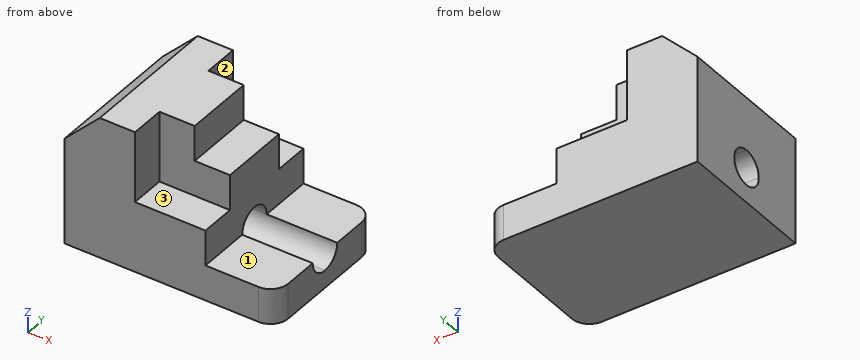
```python
from build123d import *

# Parameters (mm, degrees)
F0_W      = 76.2
F0_H      = 50.8
F1_DEPTH  = 50.8
F3_DEPTH  = 50.801
F5_DEPTH  = 12.7
F6_W      = 25.4
F6_H      = 25.4
F7_DEPTH  = 12.7
F9_DEPTH  = 12.701
F11_DEPTH = 76.201


with BuildPart() as f1:
    # F0 (on Front) → F1 (new body)
    with BuildSketch(Plane.XZ):
        with Locations((38.1, 25.4)):
            Rectangle(F0_W, F0_H)
    extrude(amount=F1_DEPTH)

    # F2 (on face) → F3 (cut, through all)
    with BuildSketch(Plane.XZ.offset(50.8)):
        Polygon((12.7, 50.8), (0, 50.8), (0, 38.1), align=None)
        Polygon((76.2, 12.7), (76.2, 50.8), (38.1, 50.8), (38.1, 38.1), (50.8, 38.1), (50.8, 12.7), align=None)
    extrude(amount=-F3_DEPTH, mode=Mode.SUBTRACT)

    # F4 (on face) → F5 (cut)
    with BuildSketch(Plane.XZ.offset(50.8)):
        Polygon((25.4, 50.8), (25.4, 25.4), (50.8, 25.4), (50.8, 38.1), (38.1, 38.1), (38.1, 50.8), align=None)
    extrude(amount=-F5_DEPTH, mode=Mode.SUBTRACT)

    # F6 (on face) → F7 (cut)
    with BuildSketch(Plane(origin=(0, 0, 0), x_dir=(-1, 0, 0), z_dir=(0, 1, 0))):
        with Locations((-38.1, 38.1)):
            Rectangle(F6_W, F6_H)
    extrude(amount=-F7_DEPTH, mode=Mode.SUBTRACT)

    # F8 (on face) → F9 (cut, through all)
    with BuildSketch(Plane.XY.offset(12.7)):
        with BuildLine():
            ThreePointArc((76.2, -44.45), (74.340128, -48.940128), (69.85, -50.8))
            Line((69.85, -50.8), (76.2, -50.8))
            Line((76.2, -50.8), (76.2, -44.45))
        make_face()
        with BuildLine():
            Line((76.2, 0), (69.85, 0))
            ThreePointArc((69.85, 0), (74.340128, -1.859872), (76.2, -6.35))
            Line((76.2, -6.35), (76.2, 0))
        make_face()
    extrude(amount=-F9_DEPTH, mode=Mode.SUBTRACT)

    # F10 (on face) → F11 (cut, through all)
    with BuildSketch(Plane.YZ.offset(76.2)):
        with BuildLine():
            ThreePointArc((-25.4, 6.35), (-20.909872, 8.209872), (-19.05, 12.7))
            ThreePointArc((-19.05, 12.7), (-20.909872, 17.190128), (-25.4, 19.05))
            ThreePointArc((-25.4, 19.05), (-29.890128, 17.190128), (-31.75, 12.7))
            ThreePointArc((-31.75, 12.7), (-29.890128, 8.209872), (-25.4, 6.35))
        make_face()
    extrude(amount=-F11_DEPTH, mode=Mode.SUBTRACT)


solid = f1.part
```
The listing builds one solid part. Answer for the finished solid, in the listing's coordinates (mm). Face numbers are marked on the shaded views. A direction names the side the tool comes from. Give positions to 0.01 mm unless a question says otherwise; leave off trailing zeros. Write each loop counter-clockwise with the first axis right and the second up, starting at its lowest first coordinate (ties: lowest second). Pieces come first, ordered by that corner, then holes. Notation, with made-up numbers: (10, 79.5) - (61, 79.5) arc R10 ccw to (61, 91.5) - close; hole circle Ø2 at (46.25, 51.5). An arc over 180 degrees is marked (long way). Use one line per item in the form item = value. Start each with the question number.
1) Consider line 1 along Z through (x, y) = (47.5, -5); line 2 along Y through (x, z) = (6.5, 8.5). Determine where each line is inside the solid, lowest interval first. Write a range as from..to.
2) Find section B-B on z = 41.5. Determine the outline of the cut face in (x, y).
3) Find section A-A on x = 23.5. Determine the outline of the cut face in (y, z), plus the area to 3 significant figures.
4) Find section C-C on y = -30.5. Determine the outline of the cut face in (x, z).
5) Flat-ended cylindrical pins translate along their axes: pin 1 Ø10 at (y, z) = (-19.5, 47.5) entering from +X; pin 2 Ø9.5 at (x, y) = (58, -43.5) entering from +Z; pin 3 Ø12 at (x, y) = (54.5, -13.5) entering from +Z. Find the tip coordinate at first contact, or state that the pin passes through.
6) A tool of negligible diameter and unlimited length cuts with its end or side. For the marked faces 1, 2 and 3, from which of +Z, -Z, +X, -X, +Y, -Y can it reach the whole face along a straight path? Write none if from no direction.
7) Find section D-D on x = 58. Determine the outline of the cut face in (y, z), plus the area to 3 significant figures.
Geometry results:
q1.line_1 = 0..25.4
q1.line_2 = -50.8..-30.16, -20.64..0
q2.outline = (3.4, -50.8) - (25.4, -50.8) - (25.4, -38.1) - (38.1, -38.1) - (38.1, -12.7) - (25.4, -12.7) - (25.4, 0) - (3.4, 0) - close
q3.outline = (-50.8, 0) - (0, 0) - (0, 50.8) - (-50.8, 50.8) - close; hole circle Ø12.7 at (-25.4, 12.7)
q3.area = 2,450 mm2
q4.outline = (0, 0) - (76.2, 0) - (76.2, 8.92) - (0, 8.92) - close; (0, 16.48) - (50.8, 16.48) - (50.8, 38.1) - (38.1, 38.1) - (38.1, 50.8) - (12.7, 50.8) - (0, 38.1) - close
q5.pin_1 = 38.1
q5.pin_2 = 12.7
q5.pin_3 = 38.1
q6.face_1 = +Z, +X, +Y, -Y
q6.face_2 = +Z, +X, +Y
q6.face_3 = +Z, +X, -Y
q7.outline = (-50.8, 0) - (0, 0) - (0, 12.7) - (-19.05, 12.7) arc R6.35 cw to (-31.75, 12.7) - (-50.8, 12.7) - close
q7.area = 582 mm2
